```python
from build123d import *

# Parameters (mm, degrees)
F0_R     = 125.9579420201
F1_DEPTH = 38.1
F3_DEPTH = 38.101


with BuildPart() as f1:
    # F0 (on Top) → F1 (new body)
    with BuildSketch(Plane.XY):
        with Locations((-30.9502501041, -23.8450411707)):
            Circle(F0_R)
    extrude(amount=-F1_DEPTH)

    # F2 (on Top) → F3 (cut, through all)
    with BuildSketch(Plane.XY):
        with BuildLine():
            ThreePointArc((-6.9e-08, -2.01e-08), (22.4870883881, 13.6312603216), (35.1458480619, 36.6798223007))
            ThreePointArc((35.1458480619, 36.6798223007), (12.6587596337, 23.0485619372), (-1.05e-08, -4.28e-08))
        make_face()
        with BuildLine():
            ThreePointArc((-70.2916961239, -73.3596446013), (-47.8046076956, -59.7283842378), (-35.1458480514, -36.6798222578))
            ThreePointArc((-35.1458480539, -36.6798222983), (-57.632936472, -50.3110826452), (-70.2916961239, -73.3596446013))
        make_face()
    extrude(amount=-F3_DEPTH, mode=Mode.SUBTRACT)


solid = f1.part
```
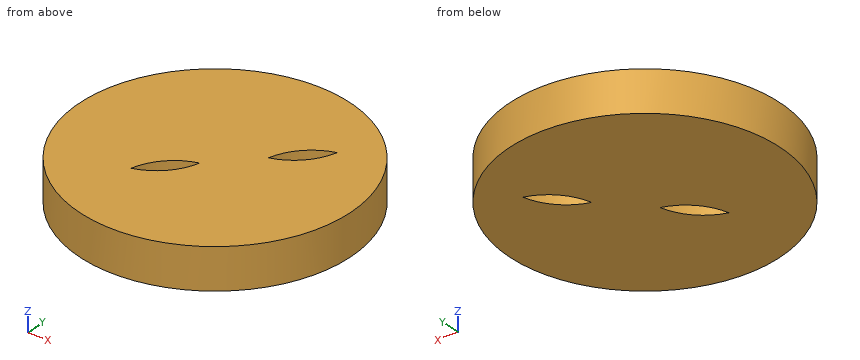
Could you check a few things on this model? Use its own coordinates, in mm. Round coordinates to 2 decimals unless told otherwise and drop trailing zeros. Order: outer loops, then holes, each group sorted by start corner. A loop starts at its lowest first (then second) coordinate and runs counter-clockwise, first axis right, second up. Notation, with made-up numbers: M 58,18 L 77,18 A25 ccw 77,44 Z; hole C 45.25,-6 d2. An arc over 180 degrees is marked long. One line per question, with ' | ' between items. Start each with the question number.
(1) Suppose I cut it at B-B on y = 25.5. List the corners of the cut face in (x, z) for me.
(2) Suppose I cut it at C-C on z = -21.5. List the corners of the cut face in (x, y) for me, then the cut area to 3 significant figures.
(3) Suppose I cut it at D-D on y = 71.5. List the corners of the cut face in (x, z) for me.
(4) For P1, Ø8, axis at y = 38.5, z = -4, coming from the -X side; P2, Ø8, axis at x = -84, z = -8.5, coming from the +Y side; P3, Ø1, axis at x = -37, z = -19, coming from the -Y side, each with a flat end and sliding along its axis, tell me the tip position at first contact or that it passes through.
(5) Please list where these lines run through material, in increasing order: line 1 along X through (y, z) = (31.5, -7.5); line 2 along X through (y, z) = (-51, -10.5); line 3 along Y through (x, z) = (15, -25).
(6) Suppose I cut it at A-A on x = -40.5. List the corners of the cut face in (y, z) for me.
Geometry results:
1) outline: M -146.84,-38.1 L 15.18,-38.1 L 15.18,0 L -146.84,0 Z; M 30.96,-38.1 L 84.94,-38.1 L 84.94,0 L 30.96,0 Z
2) outline: C -30.95,-23.85 d251.92; hole M -70.29,-73.36 A50.8 ccw -35.15,-36.68 A50.8 ccw Z; hole M 0,0 A50.8 ccw 35.15,36.68 A50.8 ccw Z | area: 48,900 mm²
3) outline: M -113.26,-38.1 L 51.36,-38.1 L 51.36,0 L -113.26,0 Z
4) P1: x = -142.58 | P2: y = 92.17 | P3: y = -149.68
5) line 1: -144.1 to 23.26, 33.58 to 82.2 | line 2: -153.95 to -58.28, -41.09 to 92.05 | line 3: -141.12 to 7.2, 25.34 to 93.43
6) outline: M -149.44,-38.1 L -50,-38.1 L -50,0 L -149.44,0 Z; M -38.57,-38.1 L 101.75,-38.1 L 101.75,0 L -38.57,0 Z
